The model under review builds one solid part; all positions refer to its coordinate system, in mm. Round coordinates to 2 decimals unless told otherwise and drop trailing zeros. Loops run counter-clockwise (first coordinate to the right, second up) from the corner with the lowest first, then second, coordinate; pieces in that order, holes last. Notation, with made-up numbers: (66.25, 69.25) -> (91.25, 69.25) arc R27 cw to (91.25, 93.25) -> close; hole circle Ø9 at (-23.75, -18.75). An arc over 180 degrees is marked (long way). Write each question's results on one line, items separated by ' | '. Start each with the question number.
Item 1: Clearance check with flat-ended pins moving along their axes: pin 1 Ø1.5 at (y, z) = (89, 1) entering from +X; pin 2 Ø1.5 at (x, z) = (322, 1) entering from -Y; pin 3 Ø1.5 at (x, z) = (160.5, 1) entering from +Y. State where each tip first meets the part, or that it passes through.
Item 2: We need section C-C (z = 1.1). Give the number of separate pieces and of enclosed holes in the cut face, and give its area (3 significant figures).
Item 3: We need section D-D (x = 23). Give the boundary of the cut face in (y, z), and give its area (3 significant figures).
Item 4: For L1, parallel to Y at x = 61.5, z = 2.35; L2, parallel to X at y = 30.5, z = 2.85; L3, parallel to X at y = 59.5, z = 1.9, list the stretches that pass through material, from the lowest coordinate up. Write a range as from..to.
Item 5: Mouldability with a two-part tool opening along X and no side actions: class faces 1 (the flat face through (159, 46, 3)), 2 (the cylindrical face through (285.346, 44.009, 1.479)) as pulls with the +X half, pulls with the -X half, needs draft (parallel to the pull), parting line crosses it, or undercut.
Item 6: We need section B-B (x = 261.5). Give the boundary of the cut face in (y, z).
Item 7: We need section A-A (y = 36.5). Give the boundary of the cut face in (x, z), and give its area (3 significant figures).
from build123d import *

# Parameters (mm, degrees)
SKETCH1_R           = 25
SKETCH1_W           = 3
SKETCH1_H           = 3
BOSS_EXTRUDE1_DEPTH = 3


with BuildPart() as part:
    # Sketch1 → Boss-Extrude1 (new body)
    with BuildSketch(Plane.XY):
        Polygon((3, 87), (3, 60), (0, 60), (0, 50), (3, 50), (3, 40), (0, 40), (0, 30), (3, 30), (3, 20), (0, 20), (0, 10), (3, 10), (3, 3), (64.6, 3), (64.6, 0), (129.2, 0), (129.2, 3), (193.8, 3), (193.8, 0), (258.4, 0), (258.4, 3), (320, 3), (320, 10), (323, 10), (323, 20), (320, 20), (320, 30), (323, 30), (323, 40), (320, 40), (320, 50), (323, 50), (323, 60), (320, 60), (320, 87), (258.4, 87), (258.4, 90), (193.8, 90), (193.8, 87), (129.2, 87), (129.2, 90), (64.6, 90), (64.6, 87), align=None)
        with Locations((61.5, 36.5)):
            Circle(SKETCH1_R, mode=Mode.SUBTRACT)
        with Locations((261.5, 36.5)):
            Circle(SKETCH1_R, mode=Mode.SUBTRACT)
        with Locations((315.5, 7.5)):
            Rectangle(SKETCH1_W, SKETCH1_H, mode=Mode.SUBTRACT)
        with Locations((7.5, 7.5)):
            Rectangle(SKETCH1_W, SKETCH1_H, mode=Mode.SUBTRACT)
    extrude(amount=BOSS_EXTRUDE1_DEPTH)


solid = part.part
Here are the results:
1) pin 1: stops at x = 258.4 | pin 2: stops at y = 10 | pin 3: stops at y = 87
2) separate pieces: 1 | enclosed holes: 4 | area: 23,600 mm2
3) outline: (3, 0) -> (87, 0) -> (87, 3) -> (3, 3) -> close | area: 252 mm2
4) L1: y = 3..11.5, 61.5..87 | L2: x = 0..37.23, 85.77..237.23, 285.77..323 | L3: x = 0..51.7, 71.3..251.7, 271.3..323
5) face 1: needs draft | face 2: undercut
6) outline: (3, 0) -> (11.5, 0) -> (11.5, 3) -> (3, 3) -> close; (61.5, 0) -> (87, 0) -> (87, 3) -> (61.5, 3) -> close
7) outline: (0, 0) -> (36.5, 0) -> (36.5, 3) -> (0, 3) -> close; (86.5, 0) -> (236.5, 0) -> (236.5, 3) -> (86.5, 3) -> close; (286.5, 0) -> (323, 0) -> (323, 3) -> (286.5, 3) -> close | area: 669 mm2
